Design review of the part built by this model. Coordinates are the model's own, in mm. Face numbers are marked on the shaded views. A direction names the side the tool comes from. Round coordinates to 2 decimals unless told otherwise and drop trailing zeros. Loops run counter-clockwise (first coordinate to the right, second up) from the corner with the lowest first, then second, coordinate; pieces in that order, holes last. Notation, with made-up numbers: (85, 41) -> (144, 41) arc R18 ccw to (144, 51) -> close; hole circle Ø10 at (57.5, 25.25). An arc over 180 degrees is marked (long way). Answer as CSV lines item,"result". Start each with the question number.
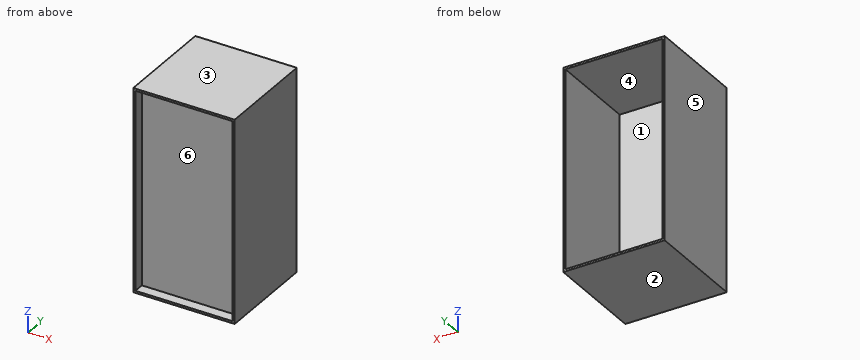
Autodesk Inventor part; units mm, degrees
ref_plane "YZ Plane" through (0, 0, 0) normal (1, 0, 0) x (0, 1, 0)
ref_plane "XZ Plane" through (0, 0, 0) normal (0, 1, 0) x (-1, 0, 0)
ref_plane "XY Plane" through (0, 0, 0) normal (0, 0, 1) x (1, 0, 0)
sketch "Sketch1" plane through (0, 0, 0) normal (0, 1, 0) x (-1, 0, 0)
  line L0 (0, 0) -> (304.8, 0)
  line L1 (304.8, 0) -> (304.8, -609.6)
  line L2 (304.8, -609.6) -> (0, -609.6)
  line L3 (0, -609.6) -> (0, 0)
  dimension "d0" = 304.8
  dimension "d1" = 609.6
extrude "Extrusion1" add sketch "Sketch1" along normal blind 304.8
sketch "Sketch2" plane through (0, 304.8, 0) normal (0, 1, 0) x (1, 0, 0)
  line L0 (-298.45, 603.25) -> (-6.35, 603.25)
  line L1 (-6.35, 603.25) -> (-6.35, 6.35)
  line L2 (-6.35, 6.35) -> (-298.45, 6.35)
  line L3 (-298.45, 6.35) -> (-298.45, 603.25)
  line L4 (0, 0) -> (0, 609.6)
  line L5 (-304.8, 609.6) -> (-304.8, 0)
  line L6 (-304.8, 0) -> (0, 0)
  line L7 (0, 609.6) -> (-304.8, 609.6)
  dimension "d4" = 6.35
  dimension "d5" = 6.35
  dimension "d6" = 6.35
  dimension "d7" = 6.35
extrude "Extrusion2" cut sketch "Sketch2" against normal blind 266.7 contours L0 L1 L2 L3
sketch "Sketch3" plane through (0, 0, 0) normal (0, -1, 0) x (1, 0, 0)
  line L0 (-298.45, -6.35) -> (-298.45, -603.25)
  line L1 (-6.35, -6.35) -> (-298.45, -6.35)
  line L2 (-298.45, -6.35) -> (-298.45, -603.25)
  line L3 (-298.45, -603.25) -> (-6.35, -603.25)
  line L4 (-6.35, -603.25) -> (-6.35, -6.35)
  line L5 (0, 0) -> (0, -609.6)
  line L6 (-304.8, 0) -> (0, 0)
  dimension "d10" = 6.35
  dimension "d11" = 6.35
extrude "Extrusion3" cut sketch "Sketch3" against normal blind 31.75
properties part number "Cargo Container"
Q1. Add section C-C, the plane x = -234.5. Give the boundary of the cut face in (y, z).
Q2. For pin 1 Ø5 at (x, z) = (-243, -188.5) entering from -Y; pin 2 Ø3 at (x, z) = (-191.5, -496) entering from +Y, all flat-tipped, find the tip position at first contact; note any pin that passes through.
Q3. Add section B-B, the plane z = -314.5. Give the boundary of the cut face in (x, y).
Q4. Add section A-A, the plane y = 114.5. Give the boundary of the cut face in (x, z), and give its area (3 significant figures).
Q5. To check wall thickness, follow probe 1 along Z at (x, y) = (-40.5, 220); probe 2 along X at (y, z) = (136.5, -149.5); probe 3 along Y at (x, z) = (-217, -400). State the ranges of each line that lie inside material, in increasing order. Write a range as from..to.
Q6. Machinability: for the marked faces 4, 5 and 6, which of the approach directions +Z, -Z, +X, -X, +Y, -Y give a long, thin tool a straight path to every point of the face, cutting with its end or side? Answer none if there is none.
Q7. Mouldability with a two-part tool opening along Z and no side actions: class the marked faces 1, 2 and 3 as pulls with the +Z half, pulls with the -Z half, needs draft (parallel to the pull), parting line crosses it, or undercut.
Worked answers:
1,outline,"(0, -609.6) -> (304.8, -609.6) -> (304.8, -603.25) -> (38.1, -603.25) -> (38.1, -6.35) -> (304.8, -6.35) -> (304.8, 0) -> (0, 0) -> (0, -6.35) -> (31.75, -6.35) -> (31.75, -603.25) -> (0, -603.25) -> close"
2,pin 1,"stops at y = 31.75"
2,pin 2,"stops at y = 38.1"
3,outline,"(-304.8, 0) -> (-298.45, 0) -> (-298.45, 31.75) -> (-6.35, 31.75) -> (-6.35, 0) -> (0, 0) -> (0, 304.8) -> (-6.35, 304.8) -> (-6.35, 38.1) -> (-298.45, 38.1) -> (-298.45, 304.8) -> (-304.8, 304.8) -> close"
4,outline,"(-304.8, -609.6) -> (0, -609.6) -> (0, 0) -> (-304.8, 0) -> close; hole (-298.45, -603.25) -> (-6.35, -603.25) -> (-6.35, -6.35) -> (-298.45, -6.35) -> close"
4,area,"11,500 mm^2"
5,probe 1,"z = -609.6..-603.25, -6.35..0"
5,probe 2,"x = -304.8..-298.45, -6.35..0"
5,probe 3,"y = 31.75..38.1"
6,face 4,"+Y"
6,face 5,"+Z, -Z, -X, +Y, -Y"
6,face 6,"-Y"
7,face 1,"undercut"
7,face 2,"pulls with the -Z half"
7,face 3,"pulls with the +Z half"
